The listing builds one solid part. Answer for the finished solid, in the listing's coordinates (mm). A direction names the side the tool comes from. Coordinates: 2 decimals unless noted, no trailing zeros. Loops run counter-clockwise (first coordinate to the right, second up) from the corner with the lowest first, then second, coordinate; pieces in that order, holes last. Notation, with made-up numbers: M -17.75,60 L 16.25,60 A21 cw 16.25,94 Z; hole C -30.5,39.25 d4. An arc over 180 degrees is marked long. Answer as a JSON object with one key per item and string values. Group by question number.
1. Straight lines are drawn through the part: L1, parallel to X at y = 2.45, z = -4; L2, parallel to X at y = 1.15, z = 4; L3, parallel to Z at x = -5, y = 1.65. For each, find the intervals that lie inside material, in ascending order.
2. Determine the mould class of faces 1 (the face through (-2.1, 1.48, -4.71)), 2 (the face through (0, 3, 0)), 3 (the face through (0.27, 1.48, -5.15)) for opening direction Z: released by +Z, released by -Z, zero draft, split by the parting line, or undercut.
3. Given pin 1 (1.3 mm diameter, centred on x = -4.5, y = 1.5, fed in from -Z); pin 2 (1.2 mm diameter, centred on x = -5, y = 1.5, fed in from +Z); pin 3 (1.2 mm diameter, centred on y = 1.5, z = 5, fed in from +X), each flat-ended and moving along its own axis, determine where each tip first touches the part or whether it passes through.
4. A cutting plane is placed at B-B on z = 3.5. Give the vertices of the cut face in (x, y), and give its area (3 significant figures).
5. A cutting plane is placed at A-A on x = 3.5. Give the vertices of the cut face in (y, z).
6. For faces 4 (the face through (-5.14, 1.48, 0.16)), 5 (the face through (5.15, 1.48, 0.27)), 6 (the face through (-4.063, 1.479, 3.145)), determine the directions among +Z, -Z, +X, -X, +Y, -Y from which every point of the face is accessible in a straight line to the end or side of a thin tool.
from build123d import *

# Parameters (mm, degrees)
Y_KSEKLIK_EKSTR_ZYON1_DEPTH = 3


with BuildPart() as part:
    # Çizim1 → Yükseklik-Ekstrüzyon1 (new body)
    with BuildSketch(Plane(origin=(0, 0, 0), x_dir=(1, 0, 0), z_dir=(0, 1, 0))):
        with BuildLine():
            Line((-1.336008246, 4.436405178), (-2.146846221, 5.247243153))
            ThreePointArc((-2.146846221, 5.247243153), (-2.164173955, 5.240120274), (-2.181478058, 5.232940176))
            Line((-2.181478058, 5.232940176), (-2.013566438, 4.172787933))
            Line((-2.013566438, 4.172787933), (-2.941264657, 4.846800142))
            ThreePointArc((-2.941264657, 4.846800142), (-2.957264794, 4.837054303), (-2.97323264, 4.827255646))
            Line((-2.97323264, 4.827255646), (-2.641543942, 3.806422801))
            Line((-2.641543942, 3.806422801), (-3.663259395, 4.327012826))
            ThreePointArc((-3.663259395, 4.327012826), (-3.67753796, 4.314884002), (-3.691776367, 4.302708061))
            Line((-3.691776367, 4.302708061), (-3.204477867, 3.346330906))
            Line((-3.204477867, 3.346330906), (-4.29505253, 3.700680094))
            ThreePointArc((-4.29505253, 3.700680094), (-4.307257936, 3.686466936), (-4.319416307, 3.672213524))
            Line((-4.319416307, 3.672213524), (-3.688506912, 2.803841239))
            Line((-3.688506912, 2.803841239), (-4.821087217, 2.983224337))
            ThreePointArc((-4.821087217, 2.983224337), (-4.830918926, 2.96727682), (-4.840697883, 2.951296902))
            Line((-4.840697883, 2.951296902), (-4.081712675, 2.192311695))
            Line((-4.081712675, 2.192311695), (-5.228410736, 2.192311695))
            ThreePointArc((-5.228410736, 2.192311695), (-5.23562666, 2.175022501), (-5.242785411, 2.157709556))
            Line((-5.242785411, 2.157709556), (-4.374413126, 1.526800161))
            Line((-4.374413126, 1.526800161), (-5.506993431, 1.347417063))
            ThreePointArc((-5.506993431, 1.347417063), (-5.511415889, 1.329211909), (-5.515778163, 1.31099224))
            Line((-5.515778163, 1.31099224), (-4.559401008, 0.82369374))
            Line((-4.559401008, 0.82369374), (-5.649975671, 0.469344552))
            ThreePointArc((-5.649975671, 0.469344552), (-5.651495767, 0.450671709), (-5.652954151, 0.431993944))
            Line((-5.652954151, 0.431993944), (-4.632121306, 0.100305246))
            Line((-4.632121306, 0.100305246), (-5.653836759, -0.42028478))
            ThreePointArc((-5.653836759, -0.42028478), (-5.652417064, -0.438965525), (-5.650935646, -0.457641477))
            Line((-5.650935646, -0.457641477), (-4.590783403, -0.625553097))
            Line((-4.590783403, -0.625553097), (-5.518481622, -1.299565306))
            ThreePointArc((-5.518481622, -1.299565306), (-5.514157093, -1.317793971), (-5.509772351, -1.336008246))
            Line((-5.509772351, -1.336008246), (-4.436405178, -1.336008246))
            Line((-4.436405178, -1.336008246), (-5.247243153, -2.146846221))
            ThreePointArc((-5.247243153, -2.146846221), (-5.240120274, -2.164173955), (-5.232940176, -2.181478058))
            Line((-5.232940176, -2.181478058), (-4.172787933, -2.013566438))
            Line((-4.172787933, -2.013566438), (-4.846800142, -2.941264657))
            ThreePointArc((-4.846800142, -2.941264657), (-4.837054303, -2.957264794), (-4.827255646, -2.97323264))
            Line((-4.827255646, -2.97323264), (-3.806422801, -2.641543942))
            Line((-3.806422801, -2.641543942), (-4.327012826, -3.663259395))
            ThreePointArc((-4.327012826, -3.663259395), (-4.314884002, -3.67753796), (-4.302708061, -3.691776367))
            Line((-4.302708061, -3.691776367), (-3.346330906, -3.204477867))
            Line((-3.346330906, -3.204477867), (-3.700680094, -4.29505253))
            ThreePointArc((-3.700680094, -4.29505253), (-3.686466936, -4.307257936), (-3.672213524, -4.319416307))
            Line((-3.672213524, -4.319416307), (-2.803841239, -3.688506912))
            Line((-2.803841239, -3.688506912), (-2.983224337, -4.821087217))
            ThreePointArc((-2.983224337, -4.821087217), (-2.96727682, -4.830918926), (-2.951296902, -4.840697883))
            Line((-2.951296902, -4.840697883), (-2.192311695, -4.081712675))
            Line((-2.192311695, -4.081712675), (-2.192311695, -5.228410736))
            ThreePointArc((-2.192311695, -5.228410736), (-2.175022501, -5.23562666), (-2.157709556, -5.242785411))
            Line((-2.157709556, -5.242785411), (-1.526800161, -4.374413126))
            Line((-1.526800161, -4.374413126), (-1.347417063, -5.506993431))
            ThreePointArc((-1.347417063, -5.506993431), (-1.329211909, -5.511415889), (-1.31099224, -5.515778163))
            Line((-1.31099224, -5.515778163), (-0.82369374, -4.559401008))
            Line((-0.82369374, -4.559401008), (-0.469344552, -5.649975671))
            ThreePointArc((-0.469344552, -5.649975671), (-0.450671709, -5.651495767), (-0.431993944, -5.652954151))
            Line((-0.431993944, -5.652954151), (-0.100305246, -4.632121306))
            Line((-0.100305246, -4.632121306), (0.42028478, -5.653836759))
            ThreePointArc((0.42028478, -5.653836759), (0.438965525, -5.652417064), (0.457641477, -5.650935646))
            Line((0.457641477, -5.650935646), (0.625553097, -4.590783403))
            Line((0.625553097, -4.590783403), (1.299565306, -5.518481622))
            ThreePointArc((1.299565306, -5.518481622), (1.317793971, -5.514157093), (1.336008246, -5.509772351))
            Line((1.336008246, -5.509772351), (1.336008246, -4.436405178))
            Line((1.336008246, -4.436405178), (2.146846221, -5.247243153))
            ThreePointArc((2.146846221, -5.247243153), (2.164173955, -5.240120274), (2.181478058, -5.232940176))
            Line((2.181478058, -5.232940176), (2.013566438, -4.172787933))
            Line((2.013566438, -4.172787933), (2.941264657, -4.846800142))
            ThreePointArc((2.941264657, -4.846800142), (2.957264794, -4.837054303), (2.97323264, -4.827255646))
            Line((2.97323264, -4.827255646), (2.641543942, -3.806422801))
            Line((2.641543942, -3.806422801), (3.663259395, -4.327012826))
            ThreePointArc((3.663259395, -4.327012826), (3.67753796, -4.314884002), (3.691776367, -4.302708061))
            Line((3.691776367, -4.302708061), (3.204477867, -3.346330906))
            Line((3.204477867, -3.346330906), (4.29505253, -3.700680094))
            ThreePointArc((4.29505253, -3.700680094), (4.307257936, -3.686466936), (4.319416307, -3.672213524))
            Line((4.319416307, -3.672213524), (3.688506912, -2.803841239))
            Line((3.688506912, -2.803841239), (4.821087217, -2.983224337))
            ThreePointArc((4.821087217, -2.983224337), (4.830918926, -2.96727682), (4.840697883, -2.951296902))
            Line((4.840697883, -2.951296902), (4.081712675, -2.192311695))
            Line((4.081712675, -2.192311695), (5.228410736, -2.192311695))
            ThreePointArc((5.228410736, -2.192311695), (5.23562666, -2.175022501), (5.242785411, -2.157709556))
            Line((5.242785411, -2.157709556), (4.374413126, -1.526800161))
            Line((4.374413126, -1.526800161), (5.506993431, -1.347417063))
            ThreePointArc((5.506993431, -1.347417063), (5.511415889, -1.329211909), (5.515778163, -1.31099224))
            Line((5.515778163, -1.31099224), (4.559401008, -0.82369374))
            Line((4.559401008, -0.82369374), (5.649975671, -0.469344552))
            ThreePointArc((5.649975671, -0.469344552), (5.651495767, -0.450671709), (5.652954151, -0.431993944))
            Line((5.652954151, -0.431993944), (4.632121306, -0.100305246))
            Line((4.632121306, -0.100305246), (5.653836759, 0.42028478))
            ThreePointArc((5.653836759, 0.42028478), (5.652417064, 0.438965525), (5.650935646, 0.457641477))
            Line((5.650935646, 0.457641477), (4.590783403, 0.625553097))
            Line((4.590783403, 0.625553097), (5.518481622, 1.299565306))
            ThreePointArc((5.518481622, 1.299565306), (5.514157093, 1.317793971), (5.509772351, 1.336008246))
            Line((5.509772351, 1.336008246), (4.436405178, 1.336008246))
            Line((4.436405178, 1.336008246), (5.247243153, 2.146846221))
            ThreePointArc((5.247243153, 2.146846221), (5.240120274, 2.164173955), (5.232940176, 2.181478058))
            Line((5.232940176, 2.181478058), (4.172787933, 2.013566438))
            Line((4.172787933, 2.013566438), (4.846800142, 2.941264657))
            ThreePointArc((4.846800142, 2.941264657), (4.837054303, 2.957264794), (4.827255646, 2.97323264))
            Line((4.827255646, 2.97323264), (3.806422801, 2.641543942))
            Line((3.806422801, 2.641543942), (4.327012826, 3.663259395))
            ThreePointArc((4.327012826, 3.663259395), (4.314884002, 3.67753796), (4.302708061, 3.691776367))
            Line((4.302708061, 3.691776367), (3.346330906, 3.204477867))
            Line((3.346330906, 3.204477867), (3.700680094, 4.29505253))
            ThreePointArc((3.700680094, 4.29505253), (3.686466936, 4.307257936), (3.672213524, 4.319416307))
            Line((3.672213524, 4.319416307), (2.803841239, 3.688506912))
            Line((2.803841239, 3.688506912), (2.983224337, 4.821087217))
            ThreePointArc((2.983224337, 4.821087217), (2.96727682, 4.830918926), (2.951296902, 4.840697883))
            Line((2.951296902, 4.840697883), (2.192311695, 4.081712675))
            Line((2.192311695, 4.081712675), (2.192311695, 5.228410736))
            ThreePointArc((2.192311695, 5.228410736), (2.175022501, 5.23562666), (2.157709556, 5.242785411))
            Line((2.157709556, 5.242785411), (1.526800161, 4.374413126))
            Line((1.526800161, 4.374413126), (1.347417063, 5.506993431))
            ThreePointArc((1.347417063, 5.506993431), (1.329211909, 5.511415889), (1.31099224, 5.515778163))
            Line((1.31099224, 5.515778163), (0.82369374, 4.559401008))
            Line((0.82369374, 4.559401008), (0.469344552, 5.649975671))
            ThreePointArc((0.469344552, 5.649975671), (0.450671709, 5.651495767), (0.431993944, 5.652954151))
            Line((0.431993944, 5.652954151), (0.100305246, 4.632121306))
            Line((0.100305246, 4.632121306), (-0.42028478, 5.653836759))
            ThreePointArc((-0.42028478, 5.653836759), (-0.438965525, 5.652417064), (-0.457641477, 5.650935646))
            Line((-0.457641477, 5.650935646), (-0.625553097, 4.590783403))
            Line((-0.625553097, 4.590783403), (-1.299565306, 5.518481622))
            ThreePointArc((-1.299565306, 5.518481622), (-1.317793971, 5.514157093), (-1.336008246, 5.509772351))
            Line((-1.336008246, 5.509772351), (-1.336008246, 4.436405178))
        make_face()
    extrude(amount=Y_KSEKLIK_EKSTR_ZYON1_DEPTH)


solid = part.part
From the geometry:
{
 "1": {"L1": "x = -3.54 to -3.02, -2.7 to 2.85, 3.23 to 3.6", "L2": "x = -3.6 to -3.23, -2.85 to 2.7, 3.02 to 3.54", "L3": "z = -2.19 to -1.98, -1.43 to -1.05, -0.68 to -0.22, 0.09 to 0.56, 0.92 to 1.34, 1.9 to 2.14"},
 "2": {"face 1": "undercut", "face 2": "zero draft", "face 3": "released by -Z"},
 "3": {"pin 1": "stops at z = -3.7", "pin 2": "stops at z = 2.97", "pin 3": "stops at x = 2.97"},
 "4": {"outline": "M -4.24,0 L -3.93,0 L -3.93,3 L -4.24,3 Z; M -3.44,0 L 3.28,0 L 3.28,3 L -3.44,3 Z; M 3.68,0 L 4.19,0 L 4.19,3 L 3.68,3 Z", "area": "22.7 mm²"},
 "5": {"outline": "M 0,-4.19 L 3,-4.19 L 3,-3.68 L 0,-3.68 Z; M 0,-3.28 L 3,-3.28 L 3,3.44 L 0,3.44 Z; M 0,3.93 L 3,3.93 L 3,4.24 L 0,4.24 Z"},
 "6": {"face 4": "-X, +Y, -Y", "face 5": "+X, +Y, -Y", "face 6": "+Y, -Y"}
}
